Job drawing, mm, ordinate dimensions from the low corner. One solid piece. Round coordinates to 2 decimals unless told otherwise and drop trailing zeros. Order: outer loops, then holes, each group sorted by start corner. A loop starts at its lowest first (then second) coordinate and runs counter-clockwise, first axis right, second up. Notation, with made-up numbers: M 67.5,-7.5 L 89.5,-7.5 A24 cw 89.5,30.5 Z; hole C -33,-6 d6. An arc over 180 degrees is marked long. Answer as a JSON object with one key per item and string values. Group by question number.
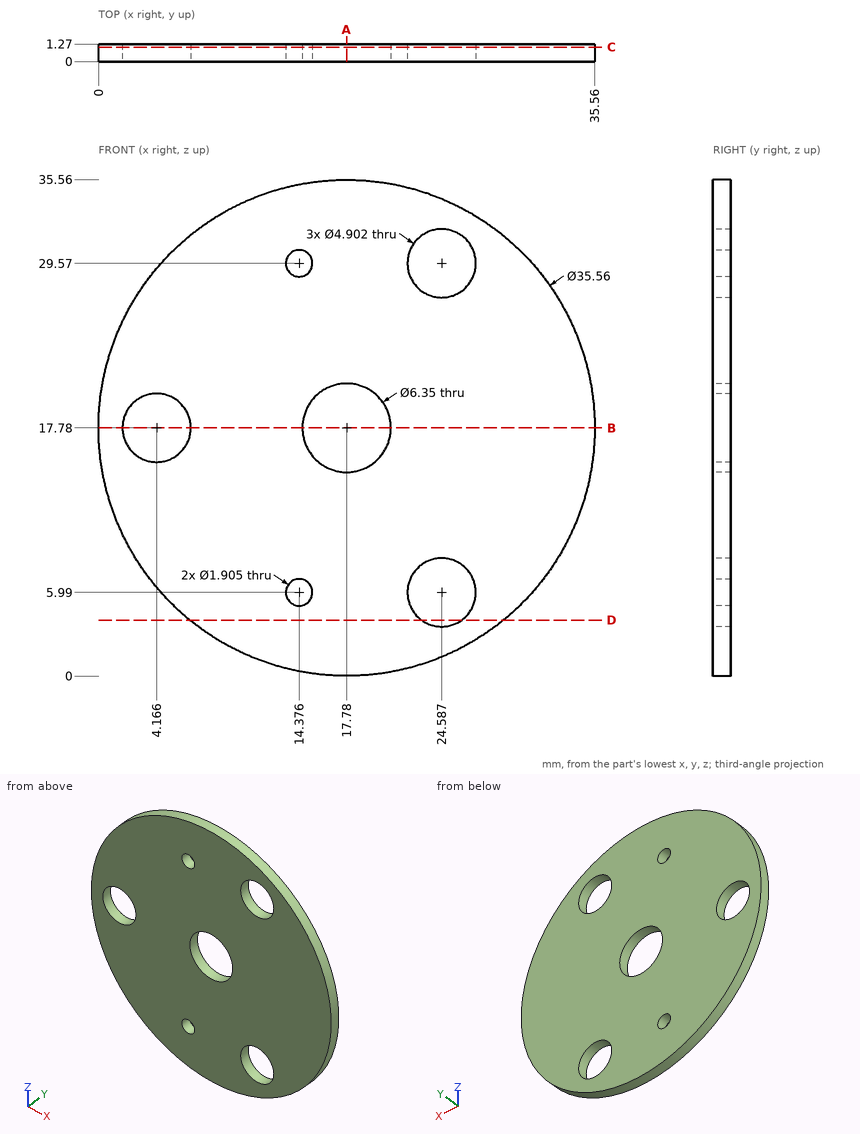
Item 1: Drill centre lines: line 1 (X direction, y = 0.6, z = 30) (1 decimal); line 2 (Z direction, x = 24, y = 0.35); line 3 (Z direction, x = 23.5, y = 0.9) (1 decimal). Where is each one in solid material? Low to high. Write a range as [from, to].
Item 2: Cut at A-A, the plane x = 17.78. Give the cut face in (y, z) (1 decimal).
Item 3: Cut at C-C, the plane y = 1.05. Give the number of separate pieces and of enclosed holes in the cut face, and give its area (3 significant figures).
Item 4: Cut at D-D, the plane z = 4. Give the cut face in (x, y) (1 decimal).
Item 5: Flat gauge pin, fed straight in: pin 1 Ø1.7 at (x, z) = (14.38, 5.99) entering from +Y. Where does the tip first touch, or does it go through?
Item 6: Cut at B-B, the plane z = 17.78. Give the cut face in (x, y) (1 decimal).
Response values:
{
 "1": {"line 1": "[4.9, 13.5], [15.2, 22.2], [27, 30.7]", "line 2": "[1.12, 3.61], [8.37, 27.19], [31.95, 34.44]", "line 3": "[0.9, 3.8], [8.2, 27.4], [31.8, 34.6]"},
 "2": {"outline": "M 0,0 L 1.3,0 L 1.3,14.6 L 0,14.6 Z; M 0,21 L 1.3,21 L 1.3,35.6 L 0,35.6 Z"},
 "3": {"separate pieces": "1", "enclosed holes": "6", "area": "899 mm^2"},
 "4": {"outline": "M 6.5,0 L 23.2,0 L 23.2,1.3 L 6.5,1.3 Z; M 26,0 L 29,0 L 29,1.3 L 26,1.3 Z"},
 "5": {"pin 1": "through"},
 "6": {"outline": "M 0,0 L 1.7,0 L 1.7,1.3 L 0,1.3 Z; M 6.6,0 L 14.6,0 L 14.6,1.3 L 6.6,1.3 Z; M 21,0 L 35.6,0 L 35.6,1.3 L 21,1.3 Z"}
}
